Autodesk Inventor part; units mm, degrees
ref_plane "YZ Plane" through (0, 0, 0) normal (1, 0, 0) x (0, 1, 0)
ref_plane "XZ Plane" through (0, 0, 0) normal (0, 1, 0) x (-1, 0, 0)
ref_plane "XY Plane" through (0, 0, 0) normal (0, 0, 1) x (1, 0, 0)
sketch "Sketch1" plane through (0, 0, 0) normal (0, 1, 0) x (-1, 0, 0)
  line L0 (12.7, -12.7) -> (-12.7, -12.7)
  line L1 (-12.7, -12.7) -> (-12.7, 12.7)
  line L2 (-12.7, 12.7) -> (12.7, 12.7)
  line L3 (12.7, 12.7) -> (12.7, -12.7)
  line L4 (-11.1125, -11.1125) -> (11.1125, -11.1125)
  line L5 (11.1125, -11.1125) -> (11.1125, 11.1125)
  line L6 (11.1125, 11.1125) -> (-11.1125, 11.1125)
  line L7 (-11.1125, 11.1125) -> (-11.1125, -11.1125)
  point P0 (0, 0)
  point P1 (0, -12.7)
  point P2 (-12.7, 0)
  dimension "d0" = 25.4
  dimension "d1" = 1.5875
extrude "Extrusion1" add sketch "Sketch1" along normal blind 1168.4
sketch "Sketch3" plane through (-12.7, 0, 12.7) normal (-1, 0, 0) x (0, 0, 1)
  arc A0 (-169.799, 314.325) -> (-166.624, 311.15) centre (-166.624, 314.325) ccw construction
  line L0 (-166.624, 311.15) -> (4.826, 311.15) construction
  arc A1 (4.826, 311.15) -> (8.001, 314.325) centre (4.826, 314.325) ccw construction
  line L1 (8.001, 314.325) -> (8.001, 442.976) construction
  arc A2 (8.001, 442.976) -> (4.826, 446.151) centre (4.826, 442.976) ccw construction
  line L2 (4.826, 446.151) -> (-32.4164, 446.151) construction
  arc A3 (-32.4164, 446.151) -> (-34.2128, 445.5939) centre (-32.4164, 442.976) ccw construction
  line L3 (-34.2128, 445.5939) -> (-168.4205, 353.498) construction
  arc A4 (-168.4205, 353.498) -> (-169.799, 350.8801) centre (-166.624, 350.8801) ccw construction
  line L4 (-169.799, 350.8801) -> (-169.799, 314.325) construction
  circle A5 centre (-12.7, 433.451) radius 3.3655
  circle A6 centre (-12.7, 382.651) radius 3.3655
  circle A7 centre (-12.7, 331.851) radius 3.3655
  circle A8 centre (-63.5, 331.851) radius 3.3655 construction
  circle A9 centre (-114.3, 331.851) radius 3.3655 construction
  circle A10 centre (-165.1, 331.851) radius 3.3655 construction
  arc A11 (-169.799, 871.474) -> (-166.624, 868.299) centre (-166.624, 871.474) ccw construction
  line L5 (-166.624, 868.299) -> (4.826, 868.299) construction
  arc A12 (4.826, 868.299) -> (8.001, 871.474) centre (4.826, 871.474) ccw construction
  line L6 (8.001, 871.474) -> (8.001, 1000.125) construction
  arc A13 (8.001, 1000.125) -> (4.826, 1003.3) centre (4.826, 1000.125) ccw construction
  line L7 (4.826, 1003.3) -> (-32.4164, 1003.3) construction
  arc A14 (-32.4164, 1003.3) -> (-34.2128, 1002.7429) centre (-32.4164, 1000.125) ccw construction
  line L8 (-34.2128, 1002.7429) -> (-168.4205, 910.647) construction
  arc A15 (-168.4205, 910.647) -> (-169.799, 908.0291) centre (-166.624, 908.0291) ccw construction
  line L9 (-169.799, 908.0291) -> (-169.799, 871.474) construction
  circle A16 centre (-12.7, 990.6) radius 3.3655
  circle A17 centre (-12.7, 939.8) radius 3.3655
  circle A18 centre (-12.7, 889) radius 3.3655
  circle A19 centre (-63.5, 889) radius 3.3655 construction
  circle A20 centre (-114.3, 889) radius 3.3655 construction
  circle A21 centre (-165.1, 889) radius 3.3655 construction
  circle A22 centre (-12.7, 1155.7) radius 3.3655
  point P0 (-12.7, 0)
  dimension "d7" = 165.1
extrude "Extrusion2" cut sketch "Sketch3" against normal blind 25.4
properties part number "Square" material "Aluminum"
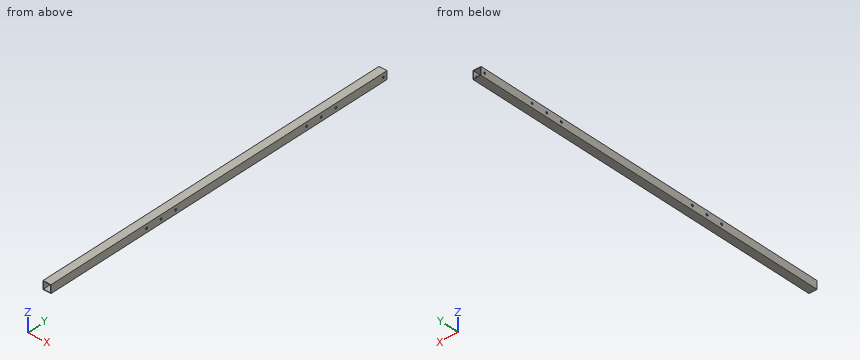
Could you check a few things on this model? Use its own coordinates, in mm. Round coordinates to 2 decimals unless told otherwise and drop trailing zeros. Write each loop counter-clockwise with the first axis right and the second up, starting at its lowest first coordinate (ties: lowest second). Pieces come first, ordered by that corner, then holes. Notation, with made-up numbers: M -24.75,47.25 L -10.75,47.25 A29 ccw -10.75,85.25 Z; hole C 54.5,-29.75 d3. An arc over 180 degrees is marked long. Answer in a Markdown table with one row per item. Add a question column.
Q1. If I drill on line 1 (X direction, y = 71, z = -1.25); line 2 (Z direction, x = 11.6, y = 1155.7), over which ranges is the centre line in solid material (lowest first)? Write a range as from..to.
Q2. Imagine slicing it at B-B (y = 109.5). Please give me the cut outline in (x, z), then the cut area to 3 significant figures.
Q3. Imagine slicing it at A-A (x = -4.75). Please give me the cut outline in (y, z).
Values:
| question | item | result |
|---|---|---|
| 1 | line 1 | -12.7..-11.11, 11.11..12.7 |
| 1 | line 2 | -12.7..-3.37, 3.37..12.7 |
| 2 | outline | M -12.7,-12.7 L 12.7,-12.7 L 12.7,12.7 L -12.7,12.7 Z; hole M -11.11,-11.11 L 11.11,-11.11 L 11.11,11.11 L -11.11,11.11 Z |
| 2 | area | 151 mm^2 |
| 3 | outline | M 0,-12.7 L 1168.4,-12.7 L 1168.4,-11.11 L 0,-11.11 Z; M 0,11.11 L 1168.4,11.11 L 1168.4,12.7 L 0,12.7 Z |
